from build123d import *

# Parameters (mm, degrees)
SKETCH1_W           = 38
SKETCH1_H           = 38
BOSS_EXTRUDE1_DEPTH = 1.5
SKETCH2_R           = 17.5
BOSS_EXTRUDE2_DEPTH = 10.7
SKETCH3_R           = 8
BOSS_EXTRUDE3_DEPTH = 3.3
SKETCH4_R           = 9.5
BOSS_EXTRUDE4_DEPTH = 11
SKETCH5_R           = 14.05
BOSS_EXTRUDE5_DEPTH = 26
SKETCH7_W           = 6
SKETCH7_H           = 21
BOSS_EXTRUDE6_DEPTH = 2.5


with BuildPart() as part:
    # Sketch1 → Boss-Extrude1 (new body)
    with BuildSketch(Plane(origin=(0, 0, 0), x_dir=(1, 0, 0), z_dir=(0, 1, 0))):
        Rectangle(SKETCH1_W, SKETCH1_H)
    extrude(amount=BOSS_EXTRUDE1_DEPTH)

    # Sketch2 → Boss-Extrude2 (add)
    with BuildSketch(Plane(origin=(0, 1.5, 0), x_dir=(1, 0, 0), z_dir=(0, 1, 0))):
        with Locations(Location((0, 0, 0), (0, 0, 270))):
            Circle(SKETCH2_R)
    extrude(amount=BOSS_EXTRUDE2_DEPTH)

    # Sketch3 → Boss-Extrude3 (add)
    with BuildSketch(Plane(origin=(0, 12.2, 0), x_dir=(1, 0, 0), z_dir=(0, 1, 0))):
        with Locations(Location((0, 0, 0), (0, 0, 270))):
            Circle(SKETCH3_R)
    extrude(amount=BOSS_EXTRUDE3_DEPTH)

    # Sketch4 → Boss-Extrude4 (add)
    with BuildSketch(Plane(origin=(0, 15.5, 0), x_dir=(1, 0, 0), z_dir=(0, 1, 0))):
        with Locations(Location((0, 0, 0), (0, 0, 270))):
            Circle(SKETCH4_R)
    extrude(amount=BOSS_EXTRUDE4_DEPTH)

    # Sketch5 → Boss-Extrude5 (add)
    with BuildSketch(Plane(origin=(0, 26.5, 0), x_dir=(1, 0, 0), z_dir=(0, 1, 0))):
        with Locations(Location((0, 0, 0), (0, 0, 90))):
            Circle(SKETCH5_R)
    extrude(amount=BOSS_EXTRUDE5_DEPTH)

    # Sketch7 → Boss-Extrude6 (add)
    with BuildSketch(Plane.XZ):
        with Locations((16, 0)):
            Rectangle(SKETCH7_W, SKETCH7_H)
    extrude(amount=BOSS_EXTRUDE6_DEPTH)


solid = part.part
Build history of the part. All positions in model axes, mm. A direction names the side the tool comes from. Coordinates: 2 decimals unless noted, no trailing zeros. Order: outer loops, then holes, each group sorted by start corner. A loop starts at its lowest first (then second) coordinate and runs counter-clockwise, first axis right, second up. Notation, with made-up numbers: M 31.5,-6 L 85.5,-6 A15 ccw 85.5,1 Z; hole C 70.25,-37 d10. An arc over 180 degrees is marked long. One line per question, with ' | ' between items. Start each with the question number.
Q1. Two-plate mould, pull along Y, no slides. Class faces 1 (the face through (-4, 12.2, 8)), 2 (the face through (-7, 15.5, -4.3)), 3 (the face through (16, -2.5, 0)), 4 (the face through (-10.648, 6.775, -13.887)): +Y half, -Y half, draft (parallel to the pull), parting line (faces both ways), or undercut.
Q2. Saw through at A-A (x = 0). List the corners of the cut face in (y, z).
Q3. Saw through at B-B (z = 0). List the corners of the cut face in (x, y), then the cut area to 3 significant figures.
Q4. 3-axis set-ups, long thin cutter, end or side, ignore diameter. For faces 5 (the face through (16, -1, -10.5)), 6 (the face through (9.2, 26.5, 3.3)), 7 (the face through (13, -1, 0)), 8 (the face through (12.465, 39.318, -6.483)), 9 (the face through (16, -1, 10.5)): which of +Z, -Z, +X, -X, +Y, -Y reach the whole face in a straight line?
Q5. Probe L1, parallel to Y at x = 10, z = -5.5; L2, parallel to Z at x = -0.5, y = 8.5; L3, parallel to Y at x = -3.5, z = -1.5. List the from-to ranges inside material, lowest first. Write a range as from..to.
Q6. Saw through at C-C (y = 19). List the corners of the cut face in (x, z).
Q7. Flat gauge pins, fed straight in: pin 1 Ø3 at (x, y) = (15.5, -1) entering from +Z; pin 2 Ø10 at (x, y) = (-7, 19) entering from -Z; pin 3 Ø3 at (x, y) = (8.5, 32.5) entering from -Z; pin 4 Ø12 at (x, y) = (8, 14) entering from -Z. Where does each tip first touch, or does it go through?
Q8. Saw through at D-D (z = 6). List the corners of the cut face in (x, y), then the cut area to 3 significant figures.
Check values:
1) face 1: undercut | face 2: undercut | face 3: -Y half | face 4: draft
2) outline: M 0,-19 L 1.5,-19 L 1.5,-17.5 L 12.2,-17.5 L 12.2,-8 L 15.5,-8 L 15.5,-9.5 L 26.5,-9.5 L 26.5,-14.05 L 52.5,-14.05 L 52.5,14.05 L 26.5,14.05 L 26.5,9.5 L 15.5,9.5 L 15.5,8 L 12.2,8 L 12.2,17.5 L 1.5,17.5 L 1.5,19 L 0,19 Z
3) outline: M -19,0 L 13,0 L 13,-2.5 L 19,-2.5 L 19,1.5 L 17.5,1.5 L 17.5,12.2 L 8,12.2 L 8,15.5 L 9.5,15.5 L 9.5,26.5 L 14.05,26.5 L 14.05,52.5 L -14.05,52.5 L -14.05,26.5 L -9.5,26.5 L -9.5,15.5 L -8,15.5 L -8,12.2 L -17.5,12.2 L -17.5,1.5 L -19,1.5 Z | area: 1,440 mm2
4) face 5: -Z, +X, -X, -Y | face 6: none | face 7: +Z, -Z, -X, -Y | face 8: +Y | face 9: +Z, +X, -X, -Y
5) L1: y = 0..12.2, 26.5..52.5 | L2: z = -17.49..17.49 | L3: y = 0..52.5
6) outline: C 0,0 d19
7) pin 1: stops at z = 19 | pin 2: stops at z = -9.29 | pin 3: stops at z = -12.18 | pin 4: stops at z = -17.35
8) outline: M -19,0 L 13,0 L 13,-2.5 L 19,-2.5 L 19,1.5 L 16.44,1.5 L 16.44,12.2 L 5.29,12.2 L 5.29,15.5 L 7.37,15.5 L 7.37,26.5 L 12.7,26.5 L 12.7,52.5 L -12.7,52.5 L -12.7,26.5 L -7.37,26.5 L -7.37,15.5 L -5.29,15.5 L -5.29,12.2 L -16.44,12.2 L -16.44,1.5 L -19,1.5 Z | area: 1,280 mm2
